Design review of the part shown in the three views and the two pictorial views. Dimensions are in mm from the part's minimum x, y and z. Coordinates: 2 decimals unless noted, no trailing zeros. Loops run counter-clockwise (first coordinate to the right, second up) from the corner with the lowest first, then second, coordinate; pieces in that order, holes last. Notation, with made-up numbers: (32, -34) -> (81, -34) arc R22 cw to (81, -11) -> close; hole circle Ø8 at (14, 66.5). An arc over 180 degrees is marked (long way). Use CSV: the item, a comma, the result in double quotes.
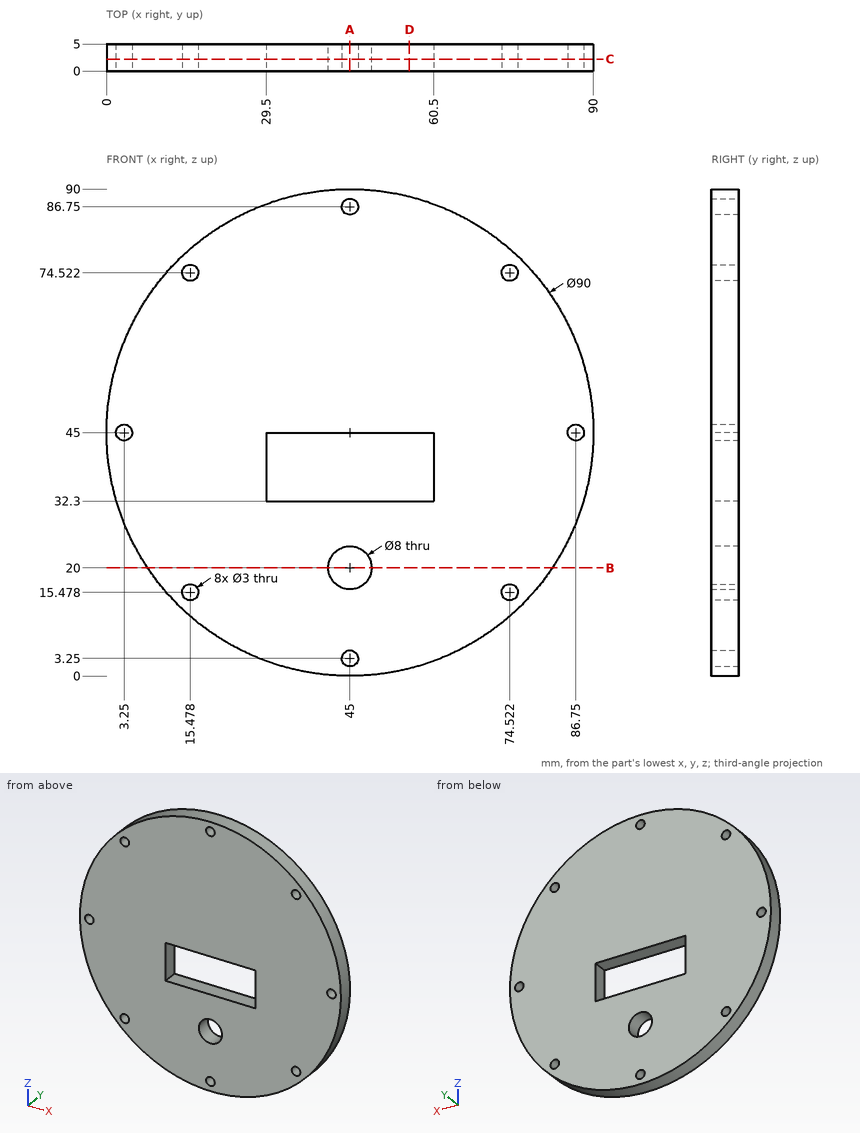
Item 1: Clearance check with flat-ended pins moving along their axes: pin 1 (2.5 mm diameter, centred on x = 45, z = 3.25, fed in from -Y); pin 2 (5 mm diameter, centred on x = 3.25, z = 45, fed in from +Y); pin 3 (2 mm diameter, centred on y = 1.5, z = 33.5, fed in from +X); pin 4 (2.5 mm diameter, centred on y = 3, z = 38, fed in from -X). State where each tip first meets the part, or that it passes through.
Checked values:
pin 1,"through"
pin 2,"y = 5"
pin 3,"x = 88.76"
pin 4,"x = 0.37"
Item 2: Add section D-D (x = 56). Give the boundary of the cut face in (y, z) (1 decimal), then the cut area to 3 significant figures.
Checked values:
outline,"(0, 1.4) -> (5, 1.4) -> (5, 32.3) -> (0, 32.3) -> close; (0, 45) -> (5, 45) -> (5, 88.6) -> (0, 88.6) -> close"
area,"373 mm^2"
Item 3: Add section C-C (y = 2.2). State how many separate pieces and enclosed holes the cut face has, then the cut area to 3 significant figures.
Checked values:
separate pieces,"1"
enclosed holes,"10"
area,"5,860 mm^2"
Item 4: To check wall thickness, follow line 1 along Z through (x, y) = (15.5, 0.4); line 2 along Z through (x, y) = (40, 1.35); line 3 along Z through (x, y) = (46, 4.75). State the ranges of each line that lie inside material, in increasing order.
Checked values:
line 1,"11.02 to 13.98, 16.98 to 73.02, 76.02 to 78.98"
line 2,"0.28 to 32.3, 45 to 89.72"
line 3,"0.01 to 2.13, 4.37 to 16.13, 23.87 to 32.3, 45 to 85.63, 87.87 to 89.99"
Item 5: Add section B-B (z = 20). Give the boundary of the cut face in (x, y).
Checked values:
outline,"(7.58, 0) -> (41, 0) -> (41, 5) -> (7.58, 5) -> close; (49, 0) -> (82.42, 0) -> (82.42, 5) -> (49, 5) -> close"
Item 6: Add section A-A (x = 45). Give the boundary of the cut face in (y, z).
Checked values:
outline,"(0, 0) -> (5, 0) -> (5, 1.75) -> (0, 1.75) -> close; (0, 4.75) -> (5, 4.75) -> (5, 16) -> (0, 16) -> close; (0, 24) -> (5, 24) -> (5, 32.3) -> (0, 32.3) -> close; (0, 45) -> (5, 45) -> (5, 85.25) -> (0, 85.25) -> close; (0, 88.25) -> (5, 88.25) -> (5, 90) -> (0, 90) -> close"
